Geometry check sheet. Reference: the model listing, model coordinates, mm. A direction names the side the tool comes from. Give positions to 0.01 mm unless a question says otherwise; leave off trailing zeros. Loops run counter-clockwise (first coordinate to the right, second up) from the corner with the lowest first, then second, coordinate; pieces in that order, holes last. Notation, with made-up numbers: (70, 87.25) -> (85, 87.25) arc R27 cw to (85, 122.25) -> close; hole circle Ø4 at (-19.75, 38). An arc over 180 degrees is marked (long way). Answer as a JSON object with one key per item and string values.
from build123d import *

# Parameters (mm, degrees)
SKETCH_R  = 0.8
PAD_DEPTH = 1.5


with BuildPart() as part:
    # Sketch → Pad (new body)
    with BuildSketch(Plane.XY):
        with BuildLine():
            Line((0, 0), (11, 0))
            Line((11, 0), (11, 4.6))
            Line((11, 4.6), (11.256218, 5.043782))
            ThreePointArc((11.256218, 5.043782), (11.286188, 5.271428), (11.14641, 5.45359))
            Line((11.14641, 5.45359), (10.2, 6))
            Line((10.2, 6), (10.2, 13.8))
            Line((10.2, 13.8), (0, 13.8))
            Line((0, 13.8), (0, 0))
        make_face()
        with Locations((5.05, 1.3)):
            Circle(SKETCH_R, mode=Mode.SUBTRACT)
        with Locations((9.7, 3.6)):
            Circle(SKETCH_R, mode=Mode.SUBTRACT)
        with Locations((3, 11.1)):
            Circle(SKETCH_R, mode=Mode.SUBTRACT)
    extrude(amount=PAD_DEPTH)


solid = part.part
1) Section check D-D on y = 7. Record the cut outline in (x, z), plus the area to 3 significant figures.
Geometry check:
{"outline": "(0, 0) -> (10.2, 0) -> (10.2, 1.5) -> (0, 1.5) -> close", "area": "15.3 mm2"}
2) Draft check along X on faces 3 (the face through (10.2, 10, 1)), 4 (the face through (3.37, 10.39, 0.74)), 5 (the face through (5, 13.8, 1)). Enter one of: pulls with the +X half, pulls with the -X half, needs draft (parallel to the pull), parting line crosses it, or undercut.
Geometry check:
{"face 3": "pulls with the +X half", "face 4": "undercut", "face 5": "needs draft"}
3) Section check B-B on z = 0.6. Record the cut outline in (x, y).
Geometry check:
{"outline": "(0, 0) -> (11, 0) -> (11, 4.6) -> (11.26, 5.04) arc R0.3 ccw to (11.15, 5.45) -> (10.2, 6) -> (10.2, 13.8) -> (0, 13.8) -> close; hole circle Ø1.6 at (3, 11.1); hole circle Ø1.6 at (5.05, 1.3); hole circle Ø1.6 at (9.7, 3.6)"}
4) Section check A-A on x = 3. Record the cut outline in (y, z).
Geometry check:
{"outline": "(0, 0) -> (10.3, 0) -> (10.3, 1.5) -> (0, 1.5) -> close; (11.9, 0) -> (13.8, 0) -> (13.8, 1.5) -> (11.9, 1.5) -> close"}
5) Section check C-C on y = 1.3. Record the cut outline in (x, z).
Geometry check:
{"outline": "(0, 0) -> (4.25, 0) -> (4.25, 1.5) -> (0, 1.5) -> close; (5.85, 0) -> (11, 0) -> (11, 1.5) -> (5.85, 1.5) -> close"}
6) Tool access check on faces 1 (the face through (11, 2, 1)), 2 (the face through (10.68, 5.723, 0.74)). Record the directions out of +Z, -Z, +X, -X, +Y, -Y that give a thin tool (end or side, any length) a straight path to the whole face; none if there is none.
Geometry check:
{"face 1": "+Z, -Z, +X, -Y", "face 2": "+Z, -Z, +X, +Y"}
7) Material ranges on line 1 along Y through (x, z) = (5, 0.1); line 2 along Y through (x, z) = (3, 0.5); line 3 along X through (y, z) = (1.25, 1), recorded low to high. Write a range as from..to.
Geometry check:
{"line 1": "y = 0..0.5, 2.1..13.8", "line 2": "y = 0..10.3, 11.9..13.8", "line 3": "x = 0..4.25, 5.85..11"}
